Build history of the part. All positions in model axes, mm. Coordinates: 2 decimals unless noted, no trailing zeros. Order: outer loops, then holes, each group sorted by start corner. A loop starts at its lowest first (then second) coordinate and runs counter-clockwise, first axis right, second up. Notation, with made-up numbers: (-5.5, 62) - (19.5, 62) arc R37 ccw to (19.5, 98) - close; hole circle Ø10 at (45.25, 27.25). An arc over 180 degrees is marked (long way). Return JSON: item names as keys, results as strings.
from build123d import *

# Parameters (mm, degrees)
SKETCH1_R           = 1.5
SKETCH1_R_2         = 12.5
BOSS_EXTRUDE1_DEPTH = 3.175
FILLET1_R           = 10
FILLET2_R           = 10


with BuildPart() as part:
    # Sketch1 → Boss-Extrude1 (new body)
    with BuildSketch(Plane.XY):
        Polygon((70.355493019, 0), (49.748846207, 49.748846207), (0, 70.355493019), (-49.748846207, 49.748846207), (-70.355493019, 0), (-49.748846207, -49.748846207), (0, -70.355493019), (49.748846207, -49.748846207), align=None)
        with Locations((0, 61.04)):
            Circle(SKETCH1_R, mode=Mode.SUBTRACT)
        with Locations((61.04, 0)):
            Circle(SKETCH1_R, mode=Mode.SUBTRACT)
        with Locations((0, -61.04)):
            Circle(SKETCH1_R, mode=Mode.SUBTRACT)
        with Locations((-61.04, 0)):
            Circle(SKETCH1_R, mode=Mode.SUBTRACT)
        with Locations((-28.535642772, 28.535642772)):
            Circle(SKETCH1_R_2, mode=Mode.SUBTRACT)
        with Locations((28.535642772, 28.535642772)):
            Circle(SKETCH1_R_2, mode=Mode.SUBTRACT)
        with Locations((-28.535642772, -28.535642772)):
            Circle(SKETCH1_R_2, mode=Mode.SUBTRACT)
        with Locations((28.535642772, -28.535642772)):
            Circle(SKETCH1_R_2, mode=Mode.SUBTRACT)
    extrude(amount=BOSS_EXTRUDE1_DEPTH)

    # Fillet1
    fillet1_edges = [part.edges().sort_by_distance(p)[0] for p in [
        (49.748846207, -49.748846207, 1.5875),
        (0, -70.355493019, 1.5875),
        (-49.748846207, -49.748846207, 1.5875),
        (-70.355493019, 0, 1.5875),
        (0, 70.355493019, 1.5875),
        (49.748846207, 49.748846207, 1.5875),
        (70.355493019, 0, 1.5875),
    ]]
    fillet(fillet1_edges, radius=FILLET1_R)

    # Fillet2
    fillet2_edges = [part.edges().sort_by_distance(p)[0] for p in [
        (-49.748846207, 49.748846207, 1.5875),
    ]]
    fillet(fillet2_edges, radius=FILLET2_R)


solid = part.part
1. Cut at B-B on x = 20. Give the cut face in (y, z) (3 decimals).
Check values:
{"outline": "(-62.071, 0) - (-37.668, 0) - (-37.668, 3.175) - (-62.071, 3.175) - close; (-19.404, 0) - (19.404, 0) - (19.404, 3.175) - (-19.404, 3.175) - close; (37.668, 0) - (62.071, 0) - (62.071, 3.175) - (37.668, 3.175) - close"}
2. Drop flat-ended pins along their axis: pin 1 (1 mm diameter, centred on y = 9, z = 2, fed in from +X); pin 2 (1.5 mm diameter, centred on y = 39, z = 2.5, fed in from +X). Give the stop position or say it passes through.
Check values:
{"pin 1": "x = 66.83", "pin 2": "x = 54.51"}
3. Cut at A-A on y = -18. Give the cut face in (x, z) (3 decimals).
Check values:
{"outline": "(-62.9, 0) - (-35.262, 0) - (-35.262, 3.175) - (-62.9, 3.175) - close; (-21.809, 0) - (21.809, 0) - (21.809, 3.175) - (-21.809, 3.175) - close; (35.262, 0) - (62.9, 0) - (62.9, 3.175) - (35.262, 3.175) - close"}
4. Cut at C-C on z = 1.1. State how many separate pieces and enclosed holes the cut face has, plus the area to 3 significant figures.
Check values:
{"separate pieces": "1", "enclosed holes": "8", "area": "12,000 mm²"}
5. Mould opens along Y. For faces 1 (the cylindrical face through (-16.989, -33.323, 1.565)), 2 (the flat face through (-60, -25, 2)), 3 (the flat face through (-1, 1, 3.175)), 4 (the cylindrical face through (18.616, -36.142, 1.565)) say: pulls with the +Y half, pulls with the -Y half, needs draft (parallel to the pull), parting line crosses it, or undercut.
Check values:
{"face 1": "undercut", "face 2": "pulls with the -Y half", "face 3": "needs draft", "face 4": "undercut"}
6. Probe L1, parallel to Y at x = -37, z = 2.3; L2, parallel to Y at x = 32, z = 1.8; L3, parallel to X at y = -36, z = 2.35. List the from-to ranges inside material, lowest first.
Check values:
{"L1": "-55.03 to -37.73, -19.34 to 19.34, 37.73 to 55.03", "L2": "-57.1 to -40.55, -16.53 to 16.53, 40.55 to 57.1", "L3": "-55.44 to -38.56, -18.51 to 18.51, 38.56 to 55.44"}
7. Cut at D-D on y = -53.5. Give the cut face in (x, z) (3 decimals), plus the area to 3 significant figures.
Check values:
{"outline": "(-40.693, 0) - (40.693, 0) - (40.693, 3.175) - (-40.693, 3.175) - close", "area": "258 mm²"}
